Read the model definition and answer for the solid it produces. Units are mm, in the model's axes. Face numbers are marked on the shaded views. Coordinates: 2 decimals unless noted, no trailing zeros. Write each loop counter-clockwise with the first axis right and the second up, starting at its lowest first coordinate (ties: lowest second). Pieces come first, ordered by that corner, then holes.
1) The part is cut by section A-A (y = 0). Determine the outline of the cut face in (x, z) (1 decimal), then the cut area to 3 significant figures.
2) Determine the mould class of the marked faces 1, 2 and 3 for opening direction Y: +Y half, -Y half, draft (parallel to the pull), parting line (faces both ways), or undercut.
3) The part is cut by section B-B (x = -11.5). Determine the outline of the cut face in (y, z) (1 decimal), then the cut area to 3 significant figures.
4) Each of these flat-tipped pins is pushed along its axis until it touches: pin 1 Ø3 at (x, y) = (-3.5, -5.5) entering from +Z; pin 2 Ø6 at (y, z) = (28, -27) entering from -X; pin 3 Ø2 at (y, z) = (-11.5, -29.5) entering from -X. Where does it stop, or does it pass through?
5) The part is cut by section C-C (z = -27.5). Determine the outline of the cut face in (x, y) (1 decimal).
6) Find the intervals of material crossed by line 1 (Y direction, x = 0, z = 2.65); line 2 (Z direction, x = -12.5, y = 26.5); line 3 (Y direction, x = -17, z = -34.5), in increasing order.
from build123d import *

# Parameters (mm, degrees)
SKETCH1_R           = 41.5163
BOSS_EXTRUDE1_DEPTH = 3.175
SKETCH2_R           = 39.6875
BOSS_EXTRUDE2_DEPTH = 38.1
SKETCH3_R           = 38.1
CUT_EXTRUDE1_DEPTH  = 1.5875


with BuildPart() as part:
    # Sketch1 → Boss-Extrude1 (new body)
    with BuildSketch(Plane.XY):
        Circle(SKETCH1_R)
    extrude(amount=BOSS_EXTRUDE1_DEPTH)

    # Sketch2 → Boss-Extrude2 (add)
    with BuildSketch(Plane(origin=(0, 0, 0), x_dir=(-1, 0, 0), z_dir=(0, 0, -1))):
        with Locations(Location((0, 0, 0), (0, 0, 180))):
            Circle(SKETCH2_R)
    extrude(amount=BOSS_EXTRUDE2_DEPTH)

    # Sketch3 → Cut-Extrude1 (cut)
    with BuildSketch(Plane.XY.offset(3.175)):
        Circle(SKETCH3_R)
    extrude(amount=-CUT_EXTRUDE1_DEPTH, mode=Mode.SUBTRACT)


solid = part.part
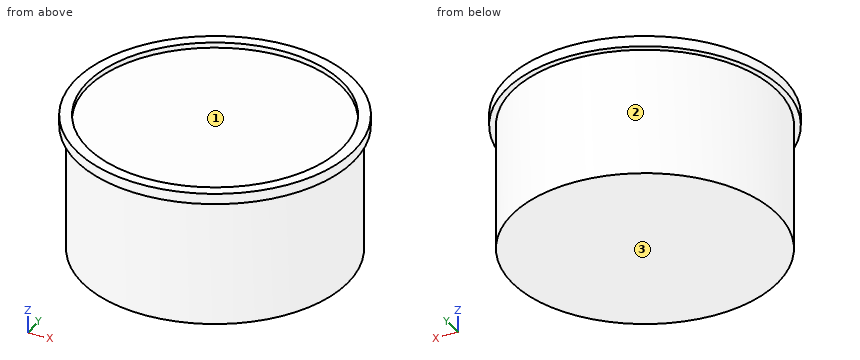
Reported:
1. outline: (-41.5, 0) - (-39.7, 0) - (-39.7, -38.1) - (39.7, -38.1) - (39.7, 0) - (41.5, 0) - (41.5, 3.2) - (38.1, 3.2) - (38.1, 1.6) - (-38.1, 1.6) - (-38.1, 3.2) - (-41.5, 3.2) - close
1. area: 3,170 mm2
2. face 1: undercut
2. face 2: parting line
2. face 3: draft
3. outline: (-39.9, 0) - (-38, 0) - (-38, -38.1) - (38, -38.1) - (38, 0) - (39.9, 0) - (39.9, 3.2) - (36.3, 3.2) - (36.3, 1.6) - (-36.3, 1.6) - (-36.3, 3.2) - (-39.9, 3.2) - close
3. area: 3,030 mm2
4. pin 1: stops at z = 1.59
4. pin 2: stops at x = -30.82
4. pin 3: stops at x = -38.27
5. outline: circle Ø79.4 at (0, 0)
6. line 1: y = -41.52 to -38.1, 38.1 to 41.52
6. line 2: z = -38.1 to 1.59
6. line 3: y = -35.86 to 35.86
